Autodesk Fusion 360 part; units mm, degrees
sketch "スケッチ1" plane through (0, 0, 0) normal (0, 0, 1) x (1, 0, 0)
  line L0 (0, 0) -> (10, 0)
  line L1 (10, 0) -> (10, 34)
  line L2 (10, 34) -> (0, 34)
  line L3 (0, 34) -> (0, 0)
  line L4 (5, 34) -> (5, 0) construction
  line L5 (0, 17) -> (10, 17) construction
  circle A0 centre (5, 17) radius 1.75
  circle A1 centre (5, 29.5) radius 1.75
  circle A2 centre (5, 4.5) radius 1.75
  dimension "d1" = 34
  dimension "d2" = 10
  dimension "d3" = 3.5
  dimension "d4" = 3.5
  dimension "d5" = 3.5
  dimension "d6" = 12.5
  dimension "d7" = 12.5
extrude "押し出し1" add sketch "スケッチ1" along normal blind 5
sketch "スケッチ2" plane through (0, 0, 5) normal (0, 0, 1) x (-1, 0, 0)
  circle A0 centre (-5, -4.5) radius 1.75
  circle A1 centre (-5, -29.5) radius 1.75
  circle A2 centre (-5, -17) radius 1.75
  line L0 (0, -34) -> (0, 0)
  line L1 (0, 0) -> (-10, 0)
  line L2 (-10, 0) -> (-10, -34)
  line L3 (-10, -34) -> (0, -34)
  circle A3 centre (-5, -29.5) radius 3
  circle A4 centre (-5, -17) radius 3
  circle A5 centre (-5, -4.5) radius 3
  dimension "d10" = 6
  dimension "d11" = 6
  dimension "d12" = 6
extrude "押し出し2" cut sketch "スケッチ2" against normal blind 3 contours A3 | A4 | A5
fillet "フィレット1" radius 1 4 edges at (0, 0, 2.5) (10, 0, 2.5) (10, 34, 2.5) (0, 34, 2.5)
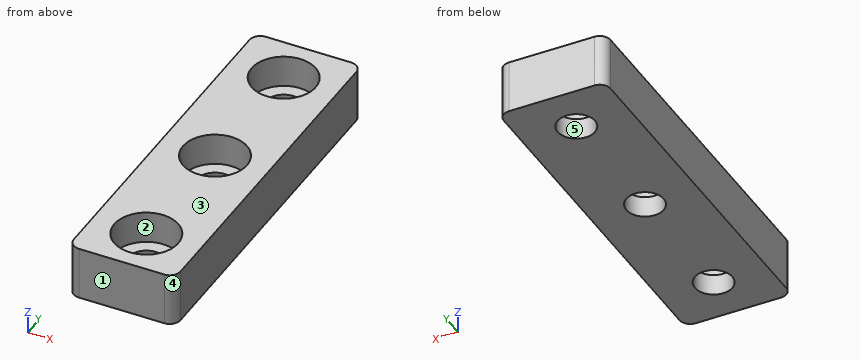
Geometry: final body of the model. Coordinates: model frame, mm. Face numbers are marked on the shaded views. A direction names the side the tool comes from. Round coordinates to 2 decimals unless told otherwise and drop trailing zeros. Order: outer loops, then holes, each group sorted by start corner. A loop starts at its lowest first (then second) coordinate and runs counter-clockwise, first axis right, second up. Notation, with made-up numbers: M 23.25,-10 L 67.25,-10 A36 ccw 67.25,29 Z; hole C 77.25,-12 d2. An arc over 180 degrees is marked long. Use one line per item in the form item = value. Start each with the question number.
Q1. Cut plane C-C (z = 1.6). Return loops of the section in (x, y).
Q2. Material intervals for line 1 (Y direction, x = 5, z = 3.15); line 2 (Y direction, x = 5, z = 1.55); line 3 (X direction, y = 17, z = 3.3), sorted ascending. Write a range as [from, to].
Q3. Cut plane A-A (y = 29.5). Return loops of the section in (x, z), and give its area (3 significant figures).
Q4. Pin query (flat end, axial travel): pin 1 Ø2 at (x, y) = (5, 4.5) entering from +Z; pin 2 Ø3 at (x, y) = (8.5, 6.5) entering from -Z; pin 3 Ø1.8 at (x, y) = (4.5, 31) entering from +Z. Return the tip coordinate at first contact, or that it passes through.
Q5. Cut plane B-B (x = 5). Return loops of the section in (y, z).
Q6. Access query for the marked faces 1 and 2. Directions: +Z, -Z, +X, -X, +Y, -Y. A direction counts if a zero-diameter tool reaches every point of the face in a straight line with its end or side. Return the directions, or none.
Q7. Mould query, pull axis X, two halves, no side actions, for the marked faces 3, 4 and 5. Classes: +X half, -X half, draft (parallel to the pull), parting line (faces both ways), or undercut.
Q8. Cut plane D-D (z = 3.55). Return loops of the section in (x, y).
Geometry results:
q1.outline = M 0,1 A1 ccw 1,0 L 9,0 A1 ccw 10,1 L 10,33 A1 ccw 9,34 L 1,34 A1 ccw 0,33 Z; hole C 5,4.5 d3.5; hole C 5,17 d3.5; hole C 5,29.5 d3.5
q2.line_1 = [0, 1.5], [7.5, 14], [20, 26.5], [32.5, 34]
q2.line_2 = [0, 2.75], [6.25, 15.25], [18.75, 27.75], [31.25, 34]
q2.line_3 = [0, 2], [8, 10]
q3.outline = M 0,0 L 3.25,0 L 3.25,2 L 2,2 L 2,5 L 0,5 Z; M 6.75,0 L 10,0 L 10,5 L 8,5 L 8,2 L 6.75,2 Z
q3.area = 25.0 mm^2
q4.pin_1 = through
q4.pin_2 = 0
q4.pin_3 = 2
q5.outline = M 0,0 L 2.75,0 L 2.75,2 L 1.5,2 L 1.5,5 L 0,5 Z; M 6.25,0 L 15.25,0 L 15.25,2 L 14,2 L 14,5 L 7.5,5 L 7.5,2 L 6.25,2 Z; M 18.75,0 L 27.75,0 L 27.75,2 L 26.5,2 L 26.5,5 L 20,5 L 20,2 L 18.75,2 Z; M 31.25,0 L 34,0 L 34,5 L 32.5,5 L 32.5,2 L 31.25,2 Z
q6.face_1 = +Z, -Z, +X, -X, -Y
q6.face_2 = +Z
q7.face_3 = draft
q7.face_4 = +X half
q7.face_5 = undercut
q8.outline = M 0,1 A1 ccw 1,0 L 9,0 A1 ccw 10,1 L 10,33 A1 ccw 9,34 L 1,34 A1 ccw 0,33 Z; hole C 5,4.5 d6; hole C 5,17 d6; hole C 5,29.5 d6
